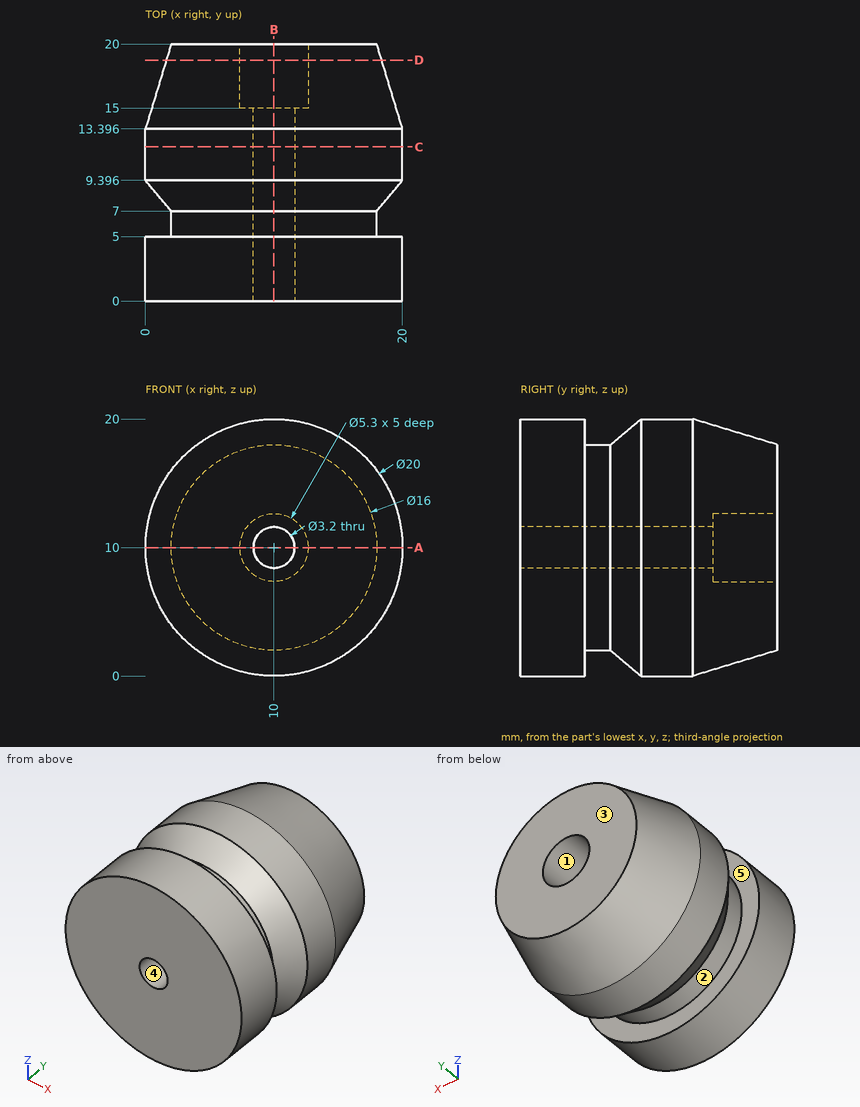
The drawing under review shows one solid part. Ordinate dimensions are in mm from its lowest x, y, z. A direction names the side the tool comes from. Give positions to 0.01 mm unless a question says otherwise; leave off trailing zeros. Write each loop counter-clockwise with the first axis right and the second up, starting at its lowest first coordinate (ties: lowest second). Pieces come first, ordered by that corner, then holes. Notation, with made-up numbers: (68, -9.5) -> (85, -9.5) arc R12 cw to (85, 5.5) -> close; hole circle Ø11 at (-34, 89). An arc over 180 degrees is marked (long way). Answer in a Markdown table with one row per item.
(1) Clearance check with flat-ended pins moving along their axes: pin 1 (4 mm diameter, centred on x = 13, y = 4, fed in from -Z); pin 2 (1 mm diameter, centred on y = 10.5, z = 13, fed in from +X); pin 3 (4 mm diameter, centred on y = 16.5, z = 5, fed in from +X). State where each tip first meets the part, or that it passes through.
Results:
| item | result |
|---|---|
| pin 1 | z = 0.05 |
| pin 2 | x = 19.68 |
| pin 3 | x = 18.79 |
(2) Consider section C-C (y = 12). State the section outline as (x, z) points, then the cut area to 3 significant figures.
Results:
| item | result |
|---|---|
| outline | circle Ø20 at (10, 10); hole circle Ø3.2 at (10, 10) |
| area | 306 mm2 |
(3) For the marked faces 4 and 5, list the 3-axis set-ups (+Z, -Z, +X, -X, +Y, -Y) from which the entire face can be reached by the end or side of a thin tool; tool diameter is ignored.
Results:
| item | result |
|---|---|
| face 4 | +Y, -Y |
| face 5 | none |
(4) To check wall thickness, follow probe 1 along X at (y, z) = (4, 10); probe 2 along Z at (x, y) = (10, 9). State the ranges of each line that lie inside material, in increasing order.
Results:
| item | result |
|---|---|
| probe 1 | 0 to 8.4, 11.6 to 20 |
| probe 2 | 0.33 to 8.4, 11.6 to 19.67 |
(5) Consider section D-D (y = 18.75). State the section outline as (x, z) points.
Results:
| item | result |
|---|---|
| outline | circle Ø16.76 at (10, 10); hole circle Ø5.3 at (10, 10) |
(6) Consider section B-B (x = 10). State the section outline as (y, z) points.
Results:
| item | result |
|---|---|
| outline | (0, 0) -> (5, 0) -> (5, 2) -> (7, 2) -> (9.4, 0) -> (13.4, 0) -> (20, 2) -> (20, 7.35) -> (15, 7.35) -> (15, 8.4) -> (0, 8.4) -> close; (0, 11.6) -> (15, 11.6) -> (15, 12.65) -> (20, 12.65) -> (20, 18) -> (13.4, 20) -> (9.4, 20) -> (7, 18) -> (5, 18) -> (5, 20) -> (0, 20) -> close |
(7) Mouldability with a two-part tool opening along X and no side actions: class the marked faces 1, 2 and 3 as +X half, -X half, draft (parallel to the pull), parting line (faces both ways), or undercut.
Results:
| item | result |
|---|---|
| face 1 | undercut |
| face 2 | parting line |
| face 3 | draft |
(8) Consider section A-A (z = 10). State the section outline as (x, y) points.
Results:
| item | result |
|---|---|
| outline | (0, 0) -> (8.4, 0) -> (8.4, 15) -> (7.35, 15) -> (7.35, 20) -> (2, 20) -> (0, 13.4) -> (0, 9.4) -> (2, 7) -> (2, 5) -> (0, 5) -> close; (11.6, 0) -> (20, 0) -> (20, 5) -> (18, 5) -> (18, 7) -> (20, 9.4) -> (20, 13.4) -> (18, 20) -> (12.65, 20) -> (12.65, 15) -> (11.6, 15) -> close |
